The figure shows three views and two pictorial views of one solid part (mm, origin at its lowest corner). Answer the questions. Round coordinates to 2 decimals unless told otherwise and drop trailing zeros. Order: outer loops, then holes, each group sorted by start corner. A loop starts at its lowest first (then second) coordinate and runs counter-clockwise, first axis right, second up. Notation, with made-up numbers: (66, 72.5) -> (91, 72.5) arc R33 ccw to (91, 110.5) -> close; hole circle Ø8 at (18, -1). An arc over 180 degrees is marked (long way). Answer in a Markdown table with one row per item. Add a question column.
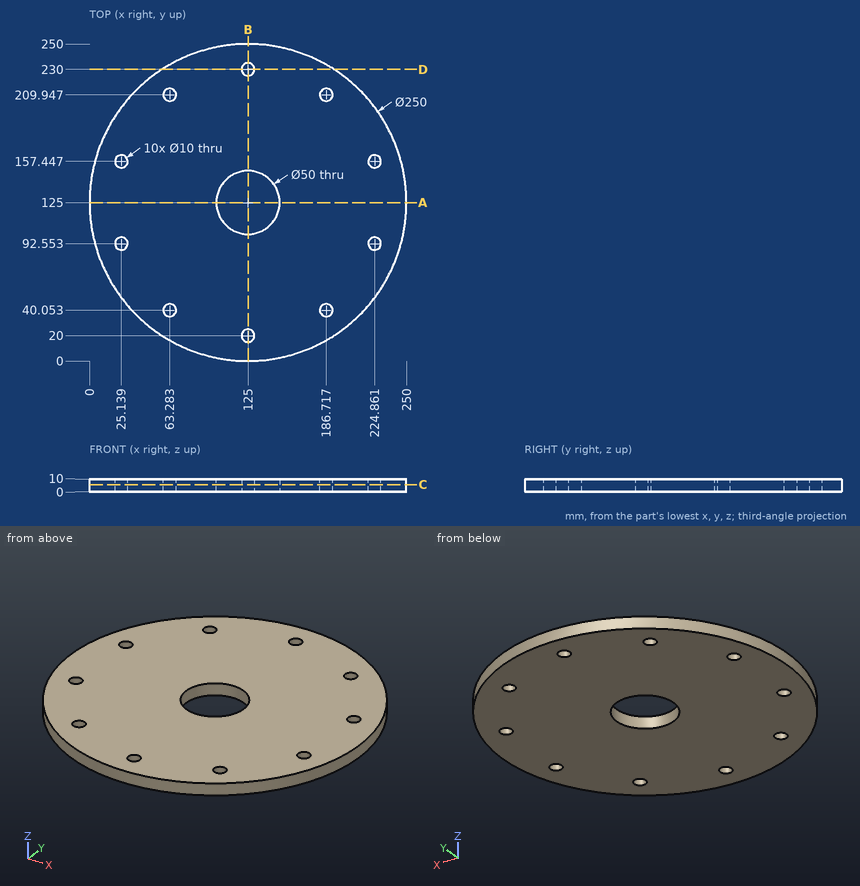
1. The part is cut by section B-B (x = 125). Give the vertices of the cut face in (y, z), then the cut area to 3 significant figures.
2. Straight lines are drawn through the part: line 1 along Y through (x, z) = (125, 3.75); line 2 along X through (y, z) = (158.5, 1.5); line 3 along Y through (x, z) = (61, 3.5) (1 decimal). For each, find the intervals that lie inside material, in ascending order.
3. The part is cut by section A-A (y = 125). Give the vertices of the cut face in (x, z), then the cut area to 3 significant figures.
4. The part is cut by section D-D (y = 230). Give the vertices of the cut face in (x, z), then the cut area to 3 significant figures.
5. The part is cut by section C-C (z = 5.5). Give the number of separate pieces and of enclosed holes in the cut face, then the cut area to 3 significant figures.
6. Each of these flat-tipped pins is pushed along its axis until it touches: pin 1 (5 mm diameter, centred on y = 27, z = 1, fed in from +X); pin 2 (8 mm diameter, centred on x = 25.14, y = 157.45, fed in from -Z); pin 3 (1 mm diameter, centred on y = 88, z = 2.5, fed in from -X); pin 4 (1.5 mm diameter, centred on x = 53.5, z = 4, fed in from +Y). Where does it stop, or does it pass through?
Report:
| question | item | result |
|---|---|---|
| 1 | outline | (0, 0) -> (15, 0) -> (15, 10) -> (0, 10) -> close; (25, 0) -> (100, 0) -> (100, 10) -> (25, 10) -> close; (150, 0) -> (225, 0) -> (225, 10) -> (150, 10) -> close; (235, 0) -> (250, 0) -> (250, 10) -> (235, 10) -> close |
| 1 | area | 1,800 mm^2 |
| 2 | line 1 | y = 0 to 15, 25 to 100, 150 to 225, 235 to 250 |
| 2 | line 2 | x = 4.57 to 20.25, 30.03 to 219.97, 229.75 to 245.43 |
| 2 | line 3 | y = 17.6 to 35.6, 44.5 to 205.5, 214.4 to 232.4 |
| 3 | outline | (0, 0) -> (100, 0) -> (100, 10) -> (0, 10) -> close; (150, 0) -> (250, 0) -> (250, 10) -> (150, 10) -> close |
| 3 | area | 2,000 mm^2 |
| 4 | outline | (57.18, 0) -> (120, 0) -> (120, 10) -> (57.18, 10) -> close; (130, 0) -> (192.82, 0) -> (192.82, 10) -> (130, 10) -> close |
| 4 | area | 1,260 mm^2 |
| 5 | separate pieces | 1 |
| 5 | enclosed holes | 11 |
| 5 | area | 46,300 mm^2 |
| 6 | pin 1 | stops at x = 205.65 |
| 6 | pin 2 | passes through |
| 6 | pin 3 | stops at x = 5.45 |
| 6 | pin 4 | stops at y = 228.05 |
